Can you work these out from the model? Positions are in its coordinate system, mm. A direction names the side the tool comes from. Coordinates: 2 decimals unless noted, no trailing zeros. Order: outer loops, then holes, each group sorted by start corner. A loop starts at its lowest first (then second) coordinate and runs counter-clockwise, first axis right, second up. Notation, with made-up numbers: (69, -36) -> (99, -36) arc R16 cw to (99, -21) -> close; hole circle Ø9 at (-19, 56). An arc over 180 degrees is marked (long way). Use a Markdown table: item, result. Add a question column.
1. For pin 1 Ø0.6 at (y, z) = (-39, 0.5) entering from +X; pin 2 Ø1 at (x, z) = (-33.5, 1) entering from -Y; pin 3 Ø1 at (y, z) = (-39.5, 1) entering from -X, each with a flat end and sliding along its axis, tell me the tip position at first contact or that it passes through.
2. If I drill on line 1 along Y through (x, z) = (33.5, 1.4), over which ranges is the centre line in solid material (lowest first)? Write a range as from..to.
3. Suppose I cut it at B-B, the plane x = -38.5. List the corners of the cut face in (y, z) for me, then the cut area to 3 significant figures.
4. For faces 1 (the flat face through (-27, -38.5, 1)), 2 (the flat face through (-1, 38.5, 1)), 3 (the flat face through (27, -38.5, 1)), which set-ups out of +Z, -Z, +X, -X, +Y, -Y let a thin tool reach every point of the face, with its end or its side?
5. Suppose I cut it at A-A, the plane z = 0.45. List the corners of the cut face in (x, y) for me, then the cut area to 3 significant figures.
```python
from build123d import *

# Parameters (mm, degrees)
SKETCH_1_W      = 91
SKETCH_1_H      = 77
SKETCH_1_W_2    = 17
SKETCH_1_H_2    = 2
EXTRUDE_1_DEPTH = 1.9


with BuildPart() as part:
    # 草图1 → 凸台-拉伸1 (new body)
    with BuildSketch(Plane.XY):
        Rectangle(SKETCH_1_W, SKETCH_1_H)
        with Locations((0, -39.5)):
            Rectangle(SKETCH_1_W_2, SKETCH_1_H_2)
    extrude(amount=EXTRUDE_1_DEPTH)


solid = part.part
```
Worked out:
| question | item | result |
|---|---|---|
| 1 | pin 1 | stops at x = 8.5 |
| 1 | pin 2 | stops at y = -38.5 |
| 1 | pin 3 | stops at x = -8.5 |
| 2 | line 1 | y = -38.5..38.5 |
| 3 | outline | (-38.5, 0) -> (38.5, 0) -> (38.5, 1.9) -> (-38.5, 1.9) -> close |
| 3 | area | 146 mm² |
| 4 | face 1 | +Z, -Z, -X, -Y |
| 4 | face 2 | +Z, -Z, +X, -X, +Y |
| 4 | face 3 | +Z, -Z, +X, -Y |
| 5 | outline | (-45.5, -38.5) -> (-8.5, -38.5) -> (-8.5, -40.5) -> (8.5, -40.5) -> (8.5, -38.5) -> (45.5, -38.5) -> (45.5, 38.5) -> (-45.5, 38.5) -> close |
| 5 | area | 7,040 mm² |
